from build123d import *

# Parameters (mm, degrees)
F1_DEPTH = 6.35
F2_DEPTH = 12.7
F4_DEPTH = 6.35
F5_R     = 5.08


with BuildPart() as f1:
    # F0 (on Top) → F1 (new body)
    with BuildSketch(Plane.XY):
        Polygon((18.330871, 10.583333), (-18.330871, 10.583333), (0, -21.166667), align=None)
        Polygon((-8.432201, 0), (-4.2161, 7.3025), (4.2161, 7.3025), (8.432201, 0), (4.2161, -7.3025), (-4.2161, -7.3025), align=None, mode=Mode.SUBTRACT)
    extrude(amount=F1_DEPTH)

    # F0 (on Top) → F2 (join)
    with BuildSketch(Plane.XY):
        Polygon((18.330871, 10.583333), (-18.330871, 10.583333), (0, -21.166667), align=None)
        Polygon((-8.432201, 0), (-4.2161, 7.3025), (4.2161, 7.3025), (8.432201, 0), (4.2161, -7.3025), (-4.2161, -7.3025), align=None, mode=Mode.SUBTRACT)
    extrude(amount=F2_DEPTH)

    # F3 (on face) → F4 (join)
    with BuildSketch(Plane(origin=(0, 0, 0), x_dir=(1, 0, 0), z_dir=(0, 0, -1))):
        Polygon((-4.2161, -7.3025), (4.2161, -7.3025), (8.432201, 0), (4.2161, 7.3025), (-4.2161, 7.3025), (-8.432201, 0), align=None)
    extrude(amount=-F4_DEPTH)

    # F5
    f5_edges = [f1.edges().sort_by_distance(p)[0] for p in [
        (18.330871, 10.583333, 6.35),
        (-18.330871, 10.583333, 6.35),
        (0, -21.166667, 6.35),
    ]]
    fillet(f5_edges, radius=F5_R)


solid = f1.part
CAD build for the part. Positions are in the model's coordinates, mm. A direction names the side the tool comes from. Round coordinates to 2 decimals unless told otherwise and drop trailing zeros. Write each loop counter-clockwise with the first axis right and the second up, starting at its lowest first coordinate (ties: lowest second). Pieces come first, ordered by that corner, then holes.
(1) 3-axis set-ups, long thin cutter, end or side, ignore diameter. For faces 1 (the face through (-6.354, 3.6, 9.481)), 2 (the face through (-13.9, 8.1, 6.4)): which of +Z, -Z, +X, -X, +Y, -Y reach the whole face in a straight line?
(2) Slice it at D-D, the plane z = 1.75. Write the cut outline in (x, y), and give its area (3 significant figures).
(3) Slice it at A-A, the plane z = 10.25. Write the cut outline in (x, y).
(4) Slice it at B-B, the plane y = 4.75. Write the cut outline in (x, z).
(5) Probe line 1 along Y through (x, z) = (-5, 7.5); line 2 along Y through (x, z) = (0.5, 7.5); line 3 along X through (y, z) = (-6.5, 7). List the from-to ranges inside material, lowest first.
(6) Drop a flat-ended pin along its axis: P1, Ø6, axis at y = -12.5, z = 10, coming from the -X side. Give the stop position or say it passes through.
(7) Slice it at C-C, the plane x = -5.5. Write the cut outline in (y, z), and give its area (3 significant figures).
(8) Mould opens along Y. For faces 3 (the face through (6.295, 3.702, 9.481)), 4 (the face through (0, 10.583, 6)), 5 (the face through (0.074, -16.086, 6.261)) say: pulls with the +Y half, pulls with the -Y half, needs draft (parallel to the pull), parting line crosses it, or undercut.
From the geometry:
1. face 1: +Z
1. face 2: +Z, -Z, -X
2. outline: (-13.93, 2.96) - (-4.4, -13.55) arc R5.08 ccw to (4.4, -13.55) - (13.93, 2.96) arc R5.08 ccw to (9.53, 10.58) - (-9.53, 10.58) arc R5.08 ccw to start
2. area: 529 mm2
3. outline: (-13.93, 2.96) - (-4.4, -13.55) arc R5.08 ccw to (4.4, -13.55) - (13.93, 2.96) arc R5.08 ccw to (9.53, 10.58) - (-9.53, 10.58) arc R5.08 ccw to start; hole (-8.43, 0) - (-4.22, -7.3) - (4.22, -7.3) - (8.43, 0) - (4.22, 7.3) - (-4.22, 7.3) - close
4. outline: (-14.56, 0) - (14.56, 0) - (14.56, 12.7) - (5.69, 12.7) - (5.69, 6.35) - (-5.69, 6.35) - (-5.69, 12.7) - (-14.56, 12.7) - close
5. line 1: y = -12.51 to -5.94, 5.94 to 10.58
5. line 2: y = -16.06 to -7.3, 7.3 to 10.58
5. line 3: x = -8.47 to -4.68, 4.68 to 8.47
6. P1: stops at x = -6.74
7. outline: (-11.64, 0) - (10.58, 0) - (10.58, 12.7) - (5.08, 12.7) - (5.08, 6.35) - (-5.08, 6.35) - (-5.08, 12.7) - (-11.64, 12.7) - close
7. area: 218 mm2
8. face 3: undercut
8. face 4: pulls with the +Y half
8. face 5: pulls with the -Y half
